Model file for the job. Use its own axes, mm. Face numbers are marked on the shaded views. A direction names the side the tool comes from. Give positions to 0.01 mm unless a question says otherwise; leave off trailing zeros. Write each loop counter-clockwise with the first axis right and the second up, starting at its lowest first coordinate (ties: lowest second). Pieces come first, ordered by that corner, then holes. Notation, with made-up numbers: M -33.75,30.5 L 25.25,30.5 A24 ccw 25.25,67.5 Z; hole C -20.5,22.5 d11. An arc over 180 degrees is marked long. Answer as a JSON object with one key per item and string values. Group by question number.
```python
from build123d import *

# Parameters (mm, degrees)
SKETCH_1_W          = 15
SKETCH_1_H          = 21.5
EXTRUDE_1_DEPTH     = 2.3
SKETCH_2_W          = 12.5
SKETCH_2_H          = 19
EXTRUDE_2_DEPTH     = 11.2
SKETCH_3_W          = 9.5
SKETCH_3_H          = 15
EXTRUDE_3_DEPTH     = 4
CUT_EXTRUDE_START   = -9.5
CUT_EXTRUDE_1_DEPTH = 9.5
SKETCH_6_W          = 3
SKETCH_6_H          = 1
EXTRUDE_1_2_DEPTH   = 7.5


# Read off the part's stored shape, not the designer's step: 切除-拉伸1
with BuildPart() as part:
    # 草图1 → Extrude 1 (new body)
    with BuildSketch(Plane.XY):
        Rectangle(SKETCH_1_W, SKETCH_1_H)
    extrude(amount=EXTRUDE_1_DEPTH)

    # 草图2 → 拉伸2 (add)
    with BuildSketch(Plane.XY.offset(2.3)):
        Rectangle(SKETCH_2_W, SKETCH_2_H)
    extrude(amount=EXTRUDE_2_DEPTH)

    # 草图3 → 拉伸3 (add)
    with BuildSketch(Plane(origin=(0, 0, 0), x_dir=(-1, 0, 0), z_dir=(0, 0, -1))):
        Rectangle(SKETCH_3_W, SKETCH_3_H)
    extrude(amount=EXTRUDE_3_DEPTH)

    # 切除-拉伸1 outline → 切除-拉伸1 (cut)
    with BuildSketch(Plane.ZY.offset(4.75).offset(CUT_EXTRUDE_START)):
        with BuildLine():
            Line((-4, -7.5), (-0.355698538, -7.5))
            add(Edge.make_bspline(
                [(-0.355698538, -7.5), (-0.354349182, -7.203584733), (-0.342893084, -4.687006069), (-0.90591647, 0.423075599), (-2.923742076, 4.765110149), (-4, 7.081043238)],
                knots=[0, 0, 0, 0, 0.058645761, 0.497905094, 1, 1, 1, 1], degree=3))
            Line((-4, 7.081043238), (-4, -7.5))
        make_face()
        with BuildLine():
            Line((-4, 7.5), (-4, 7.081043238))
            add(Edge.make_bspline(
                [(-4, 7.081043238), (-3.418318642, 7.19501669), (-2.098267317, 7.453664838), (-0.752663012, 7.483379257), (0, 7.5)],
                knots=[0, 0, 0, 0, 0.440650562, 1, 1, 1, 1], degree=3))
            Line((0, 7.5), (-4, 7.5))
        make_face()
    extrude(amount=CUT_EXTRUDE_1_DEPTH, mode=Mode.SUBTRACT)

    # 草图6 → Extrude 1 2 (add)
    with BuildSketch(Plane.XY.offset(13.5)):
        Rectangle(SKETCH_6_W, SKETCH_6_H)
        with Locations((0, 6.9)):
            Rectangle(SKETCH_6_W, SKETCH_6_H)
        with Locations((0, -6.9)):
            Rectangle(SKETCH_6_W, SKETCH_6_H)
    extrude(amount=EXTRUDE_1_2_DEPTH)


solid = part.part
```
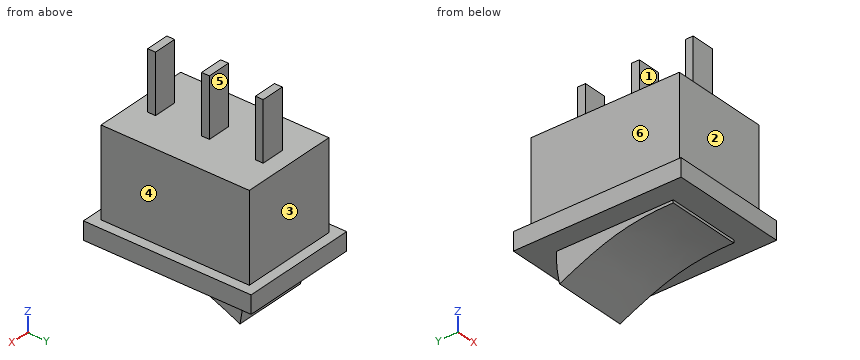
Q1. Slice it at A-A, the plane z = 16.25. Write the cut outline in (x, y), then the cut area to 3 significant figures.
Q2. Slice it at B-B, the plane y = 8.25. Write the cut outline in (x, z).
Q3. Two-plate mould, pull along Y, no slides. Class the marked faces 1, 2 and 3: +Y half, -Y half, draft (parallel to the pull), parting line (faces both ways), or undercut.
Q4. Drop flat-ended pins along their axis: P1, Ø0.8, axis at y = 0, z = 19, coming from the +X side; P2, Ø5, axis at y = 1, z = 17.5, coming from the -X side; P3, Ø1.5, axis at y = 0.5, z = 4, coming from the -X side. Give the stop position or say it passes through.
Q5. 3-axis set-ups, long thin cutter, end or side, ignore diameter. For the marked faces 4, 5 and 6: which of +Z, -Z, +X, -X, +Y, -Y reach the whole face in a straight line?
Q6. Wall check: L1, parallel to X at y = -9, z = 8.75; L2, parallel to Y at x = 2.75, z = 9.5; L3, parallel to Z at x = -5.75, y = -10. Give the ranges that are in metal, low to high.
Q7. Slice it at C-C, the plane z = 6.75. Write the cut outline in (x, y), then the cut area to 4 significant figures.
Solved:
{
 "1": {"outline": "M -1.5,-7.4 L 1.5,-7.4 L 1.5,-6.4 L -1.5,-6.4 Z; M -1.5,-0.5 L 1.5,-0.5 L 1.5,0.5 L -1.5,0.5 Z; M -1.5,6.4 L 1.5,6.4 L 1.5,7.4 L -1.5,7.4 Z", "area": "9.00 mm²"},
 "2": {"outline": "M -7.5,0 L 7.5,0 L 7.5,2.3 L 6.25,2.3 L 6.25,13.5 L -6.25,13.5 L -6.25,2.3 L -7.5,2.3 Z"},
 "3": {"face 1": "undercut", "face 2": "-Y half", "face 3": "+Y half"},
 "4": {"P1": "stops at x = 1.5", "P2": "stops at x = -1.5", "P3": "stops at x = -6.25"},
 "5": {"face 4": "+Z, +X, +Y, -Y", "face 5": "+Z, +X, -X", "face 6": "+Z, -X, +Y, -Y"},
 "6": {"L1": "x = -6.25 to 6.25", "L2": "y = -9.5 to 9.5", "L3": "z = 0 to 2.3"},
 "7": {"outline": "M -6.25,-9.5 L 6.25,-9.5 L 6.25,9.5 L -6.25,9.5 Z", "area": "237.5 mm²"}
}
